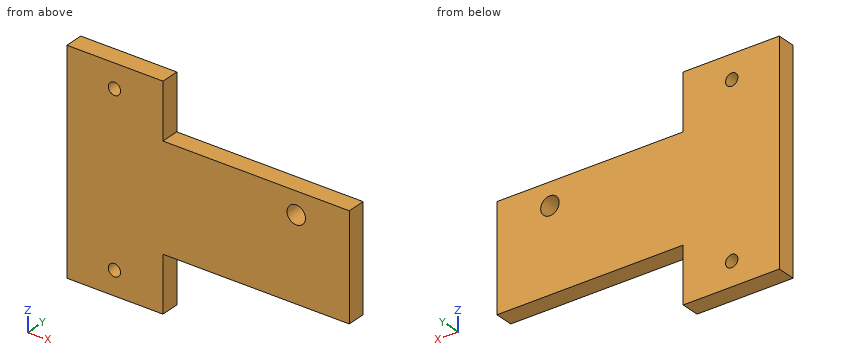
```python
from build123d import *

# Parameters (mm, degrees)
SKETCH1_W           = 46
SKETCH1_H           = 17
BOSS_EXTRUDE1_DEPTH = 3
SKETCH2_W           = 15.65
SKETCH2_H           = 3
BOSS_EXTRUDE2_DEPTH = 9
SKETCH3_R           = 1
CUT_EXTRUDE1_DEPTH  = 10
SKETCH4_R           = 1.5
CUT_EXTRUDE2_DEPTH  = 10


with BuildPart() as part:
    # Sketch1 → Boss-Extrude1 (new body)
    with BuildSketch(Plane(origin=(0, 0, 0), x_dir=(1, 0, 0), z_dir=(0, 1, 0))):
        Rectangle(SKETCH1_W, SKETCH1_H)
    extrude(amount=BOSS_EXTRUDE1_DEPTH)

    # Sketch2 → Boss-Extrude2 (add)
    with BuildSketch(Plane(origin=(0, 0, -8.5), x_dir=(-1, 0, 0), z_dir=(0, 0, -1))):
        with Locations((15.175, 1.5)):
            Rectangle(SKETCH2_W, SKETCH2_H)
    boss_extrude2 = extrude(amount=BOSS_EXTRUDE2_DEPTH)

    # Mirror1: Boss-Extrude2 across plane
    add(boss_extrude2.mirror(Plane.XY))

    # Sketch3 → Cut-Extrude1 (cut)
    with BuildSketch(Plane(origin=(0, 3, 0), x_dir=(1, 0, 0), z_dir=(0, 1, 0))):
        with Locations((-15.25, 13.625)):
            Circle(SKETCH3_R)
        with Locations((-15.25, -13.625)):
            Circle(SKETCH3_R)
    extrude(amount=-CUT_EXTRUDE1_DEPTH, mode=Mode.SUBTRACT)

    # Sketch4 → Cut-Extrude2 (cut)
    with BuildSketch(Plane(origin=(0, 3, 0), x_dir=(1, 0, 0), z_dir=(0, 1, 0))):
        with Locations((14.36, -4.9)):
            Circle(SKETCH4_R)
    extrude(amount=-CUT_EXTRUDE2_DEPTH, mode=Mode.SUBTRACT)


solid = part.part
```
Verification items for the finished model (mm, model axes). Coordinates: 2 decimals unless noted, no trailing zeros. Write each loop counter-clockwise with the first axis right and the second up, starting at its lowest first coordinate (ties: lowest second). Pieces come first, ordered by that corner, then holes. Notation, with made-up numbers: (-21, 81) - (12, 81) arc R7 ccw to (12, 89) - close; hole circle Ø6 at (9.5, -22). An arc over 180 degrees is marked (long way). One line per question, with ' | ' between items. Start each with the question number.
1. Section check D-D (y = 2.3). Enter the section's corners in (x, z) (3 decimals).
2. Material ranges on line 1 along Z through (x, y) = (-15.25, 0.8) (3 decimals); line 2 along Z through (x, y) = (14.36, 1.15); line 3 along X through (y, z) = (2.15, 4.9), recorded low to high.
3. Section check C-C (x = -15.25). Enter the section's corners in (y, z) (3 decimals).
4. Gauge pin test, flat ends, axial feed: P1, Ø2.5, axis at x = 14.36, z = 4.9, coming from the +Y side; P2, Ø1.5, axis at y = 2, z = -12, coming from the +X side; P3, Ø1.5, axis at x = 14, y = 0.5, coming from the +Z side. Record the tip position at first contact, or that the pin passes through.
5. Section check A-A (z = 4). Enter the section's corners in (x, y).
6. Section check B-B (x = 14.36). Enter the section's corners in (y, z).
Computed values:
1) outline: (-23, -17.5) - (-7.35, -17.5) - (-7.35, -8.5) - (23, -8.5) - (23, 8.5) - (-7.35, 8.5) - (-7.35, 17.5) - (-23, 17.5) - close; hole circle Ø2 at (-15.25, -13.625); hole circle Ø2 at (-15.25, 13.625); hole circle Ø3 at (14.36, 4.9)
2) line 1: -17.5 to -14.625, -12.625 to 12.625, 14.625 to 17.5 | line 2: -8.5 to 3.4, 6.4 to 8.5 | line 3: -23 to 12.86, 15.86 to 23
3) outline: (0, -17.5) - (3, -17.5) - (3, -14.625) - (0, -14.625) - close; (0, -12.625) - (3, -12.625) - (3, 12.625) - (0, 12.625) - close; (0, 14.625) - (3, 14.625) - (3, 17.5) - (0, 17.5) - close
4) P1: through | P2: x = -7.35 | P3: z = 8.5
5) outline: (-23, 0) - (13.16, 0) - (13.16, 3) - (-23, 3) - close; (15.56, 0) - (23, 0) - (23, 3) - (15.56, 3) - close
6) outline: (0, -8.5) - (3, -8.5) - (3, 3.4) - (0, 3.4) - close; (0, 6.4) - (3, 6.4) - (3, 8.5) - (0, 8.5) - close
